from build123d import *

# Parameters (mm, degrees)
SKETCH_1_R      = 18.5
SKETCH_1_R_2    = 2
SKETCH_1_R_3    = 2.08
SKETCH_1_R_4    = 8.75
EXTRUDE_1_DEPTH = 2


with BuildPart() as part:
    # 草图1 → 凸台-拉伸1 (new body)
    with BuildSketch(Plane.XY):
        with Locations((-0.985220571, 0.129022057)):
            Circle(SKETCH_1_R)
        with Locations((-0.985220571, -14.870977943)):
            Circle(SKETCH_1_R_2, mode=Mode.SUBTRACT)
        with Locations((-13.975601628, -7.370977943)):
            Circle(SKETCH_1_R_2, mode=Mode.SUBTRACT)
        with Locations((-13.975601628, 7.629022057)):
            Circle(SKETCH_1_R_2, mode=Mode.SUBTRACT)
        with Locations((-0.985220571, 15.129022057)):
            Circle(SKETCH_1_R_2, mode=Mode.SUBTRACT)
        with Locations((12.005160486, 7.629022057)):
            Circle(SKETCH_1_R_2, mode=Mode.SUBTRACT)
        with Locations((12.005160486, -7.370977943)):
            Circle(SKETCH_1_R_2, mode=Mode.SUBTRACT)
        with Locations((-14.515220571, 0.129022057)):
            Circle(SKETCH_1_R_3, mode=Mode.SUBTRACT)
        with Locations((5.779779429, 11.84634577)):
            Circle(SKETCH_1_R_3, mode=Mode.SUBTRACT)
        with Locations((5.779779429, -11.588301656)):
            Circle(SKETCH_1_R_3, mode=Mode.SUBTRACT)
        with Locations((-0.985220571, 0.129022057)):
            Circle(SKETCH_1_R_4, mode=Mode.SUBTRACT)
    extrude(amount=EXTRUDE_1_DEPTH)


solid = part.part
Work out the finished part from the listing and answer in its coordinate system (mm). Round coordinates to 2 decimals unless told otherwise and drop trailing zeros. Write each loop counter-clockwise with the first axis right and the second up, starting at its lowest first coordinate (ties: lowest second). Pieces come first, ordered by that corner, then holes. Notation, with made-up numbers: (53.5, 0.25) -> (104.5, 0.25) arc R8 cw to (104.5, 11.25) -> close; hole circle Ø3 at (-32, 49.5). An arc over 180 degrees is marked (long way). Write each question's results on one line, items separated by ' | '.
Item 1: Find the intervals of material crossed by line 1 along X through (y, z) = (-7, 0.2); line 2 along X through (y, z) = (0, 1.5); line 3 along Y through (x, z) = (7, 0.1), in increasing order. Write a range as [from, to].
Result set:
line 1: [-18.06, -15.94], [-12.01, -6.06], [4.09, 10.04], [13.97, 16.09] | line 2: [-19.48, -16.59], [-12.44, -9.73], [7.76, 17.51] | line 3: [-16.56, -13.27], [-9.9, -3.45], [3.71, 10.16], [13.53, 16.82]
Item 2: A cutting plane is placed at D-D, the plane y = -1. Determine the outline of the cut face in (x, z).
Result set:
outline: (-19.45, 0) -> (-16.26, 0) -> (-16.26, 2) -> (-19.45, 2) -> close; (-12.77, 0) -> (-9.66, 0) -> (-9.66, 2) -> (-12.77, 2) -> close; (7.69, 0) -> (17.48, 0) -> (17.48, 2) -> (7.69, 2) -> close
Item 3: A cutting plane is placed at B-B, the plane y = 3. Determine the outline of the cut face in (x, z), plus the area to 3 significant figures.
Result set:
outline: (-19.26, 0) -> (-9.25, 0) -> (-9.25, 2) -> (-19.26, 2) -> close; (7.28, 0) -> (17.29, 0) -> (17.29, 2) -> (7.28, 2) -> close | area: 40.0 mm^2
Item 4: A cutting plane is placed at A-A, the plane x = -6.5. Determine the outline of the cut face in (y, z), plus the area to 3 significant figures.
Result set:
outline: (-17.53, 0) -> (-6.66, 0) -> (-6.66, 2) -> (-17.53, 2) -> close; (6.92, 0) -> (17.79, 0) -> (17.79, 2) -> (6.92, 2) -> close | area: 43.5 mm^2
Item 5: Flat-ended cylindrical pins translate along their axes: P1, Ø1, axis at y = -5, z = 1, coming from the -X side; P2, Ø4.5, axis at x = -13.98, y = 7.63, coming from the -Z side. Find the tip coordinate at first contact, or state that the pin passes through.
Result set:
P1: x = -18.9 | P2: z = 0
Item 6: A cutting plane is placed at C-C, the plane x = -1. Determine the outline of the cut face in (y, z), plus the area to 3 significant figures.
Result set:
outline: (-18.37, 0) -> (-16.87, 0) -> (-16.87, 2) -> (-18.37, 2) -> close; (-12.87, 0) -> (-8.62, 0) -> (-8.62, 2) -> (-12.87, 2) -> close; (8.88, 0) -> (13.13, 0) -> (13.13, 2) -> (8.88, 2) -> close; (17.13, 0) -> (18.63, 0) -> (18.63, 2) -> (17.13, 2) -> close | area: 23.0 mm^2
Item 7: The mould has two halves that part along Y. Classify faces 1 (the face through (16.66, 5.69, 0.99)), 2 (the face through (3, -8, 0)), 3 (the face through (10.42, 6.41, 0.99)): +Y half, -Y half, draft (parallel to the pull), parting line (faces both ways), or undercut.
Result set:
face 1: parting line | face 2: draft | face 3: undercut
